from build123d import *

# Parameters (mm, degrees)
CUT_EXTRUDE1_DEPTH      = 304.831137641
CUT_EXTRUDE1_DEPTH_BACK = 304.831137641
SKETCH2_R               = 11.085
CUT_EXTRUDE2_DEPTH      = 304.831137641
CUT_EXTRUDE2_DEPTH_BACK = 304.831137641
FILLET1_R               = 0.146825397
SKETCH8_R               = 24.5
CUT_EXTRUDE3_DEPTH      = 9.690476191
FILLET4_R               = 0.044047619


with BuildPart() as part:
    # Sketch1 → Revolve1 (revolve)
    with BuildSketch(Plane.XY):
        with BuildLine():
            Line((34.01, 60.44), (30.5, 60.44))
            Line((30.5, 60.44), (30.5, 300))
            Line((30.5, 300), (18.5, 300))
            Line((18.5, 300), (18.5, 60.44))
            Line((18.5, 60.44), (0, 60.44))
            Line((0, 60.44), (0, 0))
            ThreePointArc((0, 0), (15.676557339, 6.493442661), (22.17, 22.17))
            Line((22.17, 22.17), (22.17, 53.2))
            Line((22.17, 53.2), (34.01, 53.2))
            Line((34.01, 53.2), (34.01, 60.44))
        make_face()
    revolve(axis=Axis((0, 0, 0), (0, 1, 0)))

    # Sketch2 → Cut-Extrude1 (cut, two sides: drawn at the far end of the back side and taken through both)
    with BuildSketch(Plane(origin=(0, 0, 0), x_dir=(0, 0, -1), z_dir=(1, 0, 0)).offset(-CUT_EXTRUDE1_DEPTH_BACK)):
        with Locations((0, 22.17)):
            Circle(SKETCH2_R)
    extrude(amount=CUT_EXTRUDE1_DEPTH + CUT_EXTRUDE1_DEPTH_BACK, mode=Mode.SUBTRACT)

    # Sketch3 → Cut-Extrude2 (cut, two sides: drawn at the far end of the back side and taken through both)
    with BuildSketch(Plane.XY.offset(-CUT_EXTRUDE2_DEPTH_BACK)):
        Polygon((-53.33, 49.26), (-53.33, 0), (-14.78, 0), (-14.78, 28.148148148), (-14.78, 49.26), (-35.888888889, 49.26), align=None)
        Polygon((35.888888889, 49.26), (53.33, 49.26), (53.33, 0), (14.78, 0), (14.78, 28.148148148), (14.78, 49.26), align=None)
    extrude(amount=CUT_EXTRUDE2_DEPTH + CUT_EXTRUDE2_DEPTH_BACK, mode=Mode.SUBTRACT)

    # Fillet1
    fillet1_edges = [part.edges().sort_by_distance(p)[0] for p in [
        (-22.17, 53.2, 0),
        (14.78, 49.26, 0),
        (-14.78, 49.26, 0),
    ]]
    fillet(fillet1_edges, radius=FILLET1_R)

    # Sketch8 → Cut-Extrude3 (cut)
    with BuildSketch(Plane(origin=(0, 300, 0), x_dir=(1, 0, 0), z_dir=(0, 1, 0))):
        with Locations(Location((0, 0, 0), (0, 0, 180))):
            Circle(SKETCH8_R)
    extrude(amount=-CUT_EXTRUDE3_DEPTH, mode=Mode.SUBTRACT)

    # Fillet4
    fillet4_edges = [part.edges().sort_by_distance(p)[0] for p in [
        (-18.5, 290.309523809, 0),
        (24.5, 300, 0),
        (-30.5, 300, 0),
    ]]
    fillet(fillet4_edges, radius=FILLET4_R)


solid = part.part
CAD build for the part. Positions are in the model's coordinates, mm. A direction names the side the tool comes from. Round coordinates to 2 decimals unless told otherwise and drop trailing zeros. Loops run counter-clockwise (first coordinate to the right, second up) from the corner with the lowest first, then second, coordinate; pieces in that order, holes last.
(1) Cut at B-B (y = 213.5). Give the cut face in (x, z), plus the area to 3 significant figures.
(2) Drop flat-ended pins along their axis: pin 1 (6 mm diameter, centred on x = 19, y = 60, fed in from -Z); pin 2 (3.5 mm diameter, centred on x = -19, z = 2, fed in from -Y); pin 3 (1 mm diameter, centred on x = 0, y = 31, fed in from -Z). Give the stop position or say it passes through.
(3) Which spindle directions (+Z, -Z, +X, -X, +Y, -Y) get a long thin tool onto all of the face, cutting with end or side? Do faces 1 (the flat face through (-14.78, 37, 0)), 2 (the flat face through (2, 300, -25)), 3 (the flat face through (-9, 290.31, 16.4)), 4 (the flat face through (-7, 53.2, 22)), 5 (the flat face through (18, 49.26, 0)). Say none if no direction does.
(4) Two-plate mould, pull along Z, no slides. Class faces 6 (the cylindrical face through (10.23, 37.83, 19.67)), 7 (the flat face through (-18, 49.26, 0)), 8 (the cylindrical face through (-13.17, 295.2, 20.66)): +Z half, -Z half, draft (parallel to the pull), parting line (faces both ways), or undercut.
(5) Wall check: line 1 along X through (y, z) = (178, -0.5); line 2 along Z through (x, y) = (0, 294). Give the ranges that are in metal, low to high.
Findings below:
1. outline: circle Ø61 at (0, 0); hole circle Ø37 at (0, 0)
1. area: 1,850 mm2
2. pin 1: stops at z = -30.01
2. pin 2: stops at y = 49.26
2. pin 3: stops at z = -22.17
3. face 1: +Z, -Z, -X, -Y
3. face 2: +Z, -Z, +X, -X, +Y
3. face 3: +Y
3. face 4: -Y
3. face 5: +Z, -Z, +X, -Y
4. face 6: parting line
4. face 7: draft
4. face 8: undercut
5. line 1: x = -30.5 to -18.49, 18.49 to 30.5
5. line 2: z = -30.5 to -24.5, 24.5 to 30.5
